```python
from build123d import *

# Parameters (mm, degrees)
SKETCH1_W           = 180
SKETCH1_H           = 180
SKETCH1_R           = 1.5
BOSS_EXTRUDE1_DEPTH = 5
CUT_EXTRUDE1_REACH  = 129.377
SKETCH4_W           = 5.1
SKETCH4_H           = 10
SKETCH4_W_2         = 10
SKETCH4_H_2         = 5.1
SKETCH4_W_3         = 125
SKETCH4_H_3         = 45
SKETCH5_R           = 1.55
CUT_EXTRUDE3_DEPTH  = 128.377392029
SKETCH6_W           = 4
SKETCH6_H           = 30
SKETCH6_R           = 1.3
CUT_EXTRUDE5_DEPTH  = 10
SKETCH7_R           = 1.55
CUT_EXTRUDE6_DEPTH  = 128.377392029
FILLET1_R           = 3


with BuildPart() as part:
    # Sketch1 → Boss-Extrude1 (new body)
    with BuildSketch(Plane(origin=(0, 0, 0), x_dir=(1, 0, 0), z_dir=(0, 1, 0))):
        Rectangle(SKETCH1_W, SKETCH1_H)
        with Locations(Location((-86, 86, 0), (0, 0, 270))):
            Circle(SKETCH1_R, mode=Mode.SUBTRACT)
        with Locations(Location((86, 86, 0), (0, 0, 270))):
            Circle(SKETCH1_R, mode=Mode.SUBTRACT)
        with Locations(Location((85.840740741, -86, 0), (0, 0, 270))):
            Circle(SKETCH1_R, mode=Mode.SUBTRACT)
        with Locations(Location((-86.159259259, -86, 0), (0, 0, 270))):
            Circle(SKETCH1_R, mode=Mode.SUBTRACT)
    extrude(amount=BOSS_EXTRUDE1_DEPTH)

    # Sketch4 → Cut-Extrude1 (cut, up to next)
    with BuildSketch(Plane(origin=(0, 5, 0), x_dir=(1, 0, 0), z_dir=(0, 1, 0)), mode=Mode.PRIVATE) as cut_extrude1_sk1:
        with Locations((67.45, -28.333333333)):
            Rectangle(SKETCH4_W, SKETCH4_H)
    cut_extrude1_tool1 = extrude(cut_extrude1_sk1.sketch, amount=-CUT_EXTRUDE1_REACH, mode=Mode.PRIVATE) & part.part
    # Sketch4 → Cut-Extrude1 (cut, up to next)
    with BuildSketch(Plane(origin=(0, 5, 0), x_dir=(1, 0, 0), z_dir=(0, 1, 0)), mode=Mode.PRIVATE) as cut_extrude1_sk2:
        with Locations((37.5, -12.55)):
            Rectangle(SKETCH4_W_2, SKETCH4_H_2)
    cut_extrude1_tool2 = extrude(cut_extrude1_sk2.sketch, amount=-CUT_EXTRUDE1_REACH, mode=Mode.PRIVATE) & part.part
    # Sketch4 → Cut-Extrude1 (cut, up to next)
    with BuildSketch(Plane(origin=(0, 5, 0), x_dir=(1, 0, 0), z_dir=(0, 1, 0)), mode=Mode.PRIVATE) as cut_extrude1_sk3:
        with Locations((0, -12.55)):
            Rectangle(SKETCH4_W_2, SKETCH4_H_2)
    cut_extrude1_tool3 = extrude(cut_extrude1_sk3.sketch, amount=-CUT_EXTRUDE1_REACH, mode=Mode.PRIVATE) & part.part
    # Sketch4 → Cut-Extrude1 (cut, up to next)
    with BuildSketch(Plane(origin=(0, 5, 0), x_dir=(1, 0, 0), z_dir=(0, 1, 0)), mode=Mode.PRIVATE) as cut_extrude1_sk4:
        with Locations((-37.5, -12.55)):
            Rectangle(SKETCH4_W_2, SKETCH4_H_2)
    cut_extrude1_tool4 = extrude(cut_extrude1_sk4.sketch, amount=-CUT_EXTRUDE1_REACH, mode=Mode.PRIVATE) & part.part
    # Sketch4 → Cut-Extrude1 (cut, up to next)
    with BuildSketch(Plane(origin=(0, 5, 0), x_dir=(1, 0, 0), z_dir=(0, 1, 0)), mode=Mode.PRIVATE) as cut_extrude1_sk5:
        with Locations((-67.45, -28.333333333)):
            Rectangle(SKETCH4_W, SKETCH4_H)
    cut_extrude1_tool5 = extrude(cut_extrude1_sk5.sketch, amount=-CUT_EXTRUDE1_REACH, mode=Mode.PRIVATE) & part.part
    # Sketch4 → Cut-Extrude1 (cut, up to next)
    with BuildSketch(Plane(origin=(0, 5, 0), x_dir=(1, 0, 0), z_dir=(0, 1, 0)), mode=Mode.PRIVATE) as cut_extrude1_sk6:
        with Locations((-37.5, -67.45)):
            Rectangle(SKETCH4_W_2, SKETCH4_H_2)
    cut_extrude1_tool6 = extrude(cut_extrude1_sk6.sketch, amount=-CUT_EXTRUDE1_REACH, mode=Mode.PRIVATE) & part.part
    # Sketch4 → Cut-Extrude1 (cut, up to next)
    with BuildSketch(Plane(origin=(0, 5, 0), x_dir=(1, 0, 0), z_dir=(0, 1, 0)), mode=Mode.PRIVATE) as cut_extrude1_sk7:
        with Locations((67.45, -51.666666667)):
            Rectangle(SKETCH4_W, SKETCH4_H)
    cut_extrude1_tool7 = extrude(cut_extrude1_sk7.sketch, amount=-CUT_EXTRUDE1_REACH, mode=Mode.PRIVATE) & part.part
    # Sketch4 → Cut-Extrude1 (cut, up to next)
    with BuildSketch(Plane(origin=(0, 5, 0), x_dir=(1, 0, 0), z_dir=(0, 1, 0)), mode=Mode.PRIVATE) as cut_extrude1_sk8:
        with Locations((37.5, -67.45)):
            Rectangle(SKETCH4_W_2, SKETCH4_H_2)
    cut_extrude1_tool8 = extrude(cut_extrude1_sk8.sketch, amount=-CUT_EXTRUDE1_REACH, mode=Mode.PRIVATE) & part.part
    # Sketch4 → Cut-Extrude1 (cut, up to next)
    with BuildSketch(Plane(origin=(0, 5, 0), x_dir=(1, 0, 0), z_dir=(0, 1, 0)), mode=Mode.PRIVATE) as cut_extrude1_sk9:
        with Locations((0, -67.45)):
            Rectangle(SKETCH4_W_2, SKETCH4_H_2)
    cut_extrude1_tool9 = extrude(cut_extrude1_sk9.sketch, amount=-CUT_EXTRUDE1_REACH, mode=Mode.PRIVATE) & part.part
    # Sketch4 → Cut-Extrude1 (cut, up to next)
    with BuildSketch(Plane(origin=(0, 5, 0), x_dir=(1, 0, 0), z_dir=(0, 1, 0)), mode=Mode.PRIVATE) as cut_extrude1_sk10:
        with Locations((-67.45, -51.666666667)):
            Rectangle(SKETCH4_W, SKETCH4_H)
    cut_extrude1_tool10 = extrude(cut_extrude1_sk10.sketch, amount=-CUT_EXTRUDE1_REACH, mode=Mode.PRIVATE) & part.part
    # Sketch4 → Cut-Extrude1 (cut, up to next)
    with BuildSketch(Plane(origin=(0, 5, 0), x_dir=(1, 0, 0), z_dir=(0, 1, 0)), mode=Mode.PRIVATE) as cut_extrude1_sk11:
        with Locations((0, -40)):
            Rectangle(SKETCH4_W_3, SKETCH4_H_3)
    cut_extrude1_tool11 = extrude(cut_extrude1_sk11.sketch, amount=-CUT_EXTRUDE1_REACH, mode=Mode.PRIVATE) & part.part
    add(cut_extrude1_tool1.solids().sort_by_distance((67.45, 5, 28.333333))[0], mode=Mode.SUBTRACT)
    add(cut_extrude1_tool2.solids().sort_by_distance((37.5, 5, 12.55))[0], mode=Mode.SUBTRACT)
    add(cut_extrude1_tool3.solids().sort_by_distance((0, 5, 12.55))[0], mode=Mode.SUBTRACT)
    add(cut_extrude1_tool4.solids().sort_by_distance((-37.5, 5, 12.55))[0], mode=Mode.SUBTRACT)
    add(cut_extrude1_tool5.solids().sort_by_distance((-67.45, 5, 28.333333))[0], mode=Mode.SUBTRACT)
    add(cut_extrude1_tool6.solids().sort_by_distance((-37.5, 5, 67.45))[0], mode=Mode.SUBTRACT)
    add(cut_extrude1_tool7.solids().sort_by_distance((67.45, 5, 51.666667))[0], mode=Mode.SUBTRACT)
    add(cut_extrude1_tool8.solids().sort_by_distance((37.5, 5, 67.45))[0], mode=Mode.SUBTRACT)
    add(cut_extrude1_tool9.solids().sort_by_distance((0, 5, 67.45))[0], mode=Mode.SUBTRACT)
    add(cut_extrude1_tool10.solids().sort_by_distance((-67.45, 5, 51.666667))[0], mode=Mode.SUBTRACT)
    add(cut_extrude1_tool11.solids().sort_by_distance((0, 5, 40))[0], mode=Mode.SUBTRACT)

    # Sketch5 → Cut-Extrude3 (cut, through all)
    with BuildSketch(Plane(origin=(0, 5, 0), x_dir=(1, 0, 0), z_dir=(0, 1, 0))):
        with Locations(Location((-47, 52, 0), (0, 0, 270))):
            Circle(SKETCH5_R)
        with Locations(Location((-23, 52, 0), (0, 0, 270))):
            Circle(SKETCH5_R)
        with Locations(Location((-23, 28, 0), (0, 0, 270))):
            Circle(SKETCH5_R)
        with Locations(Location((-47, 28, 0), (0, 0, 270))):
            Circle(SKETCH5_R)
    extrude(amount=-CUT_EXTRUDE3_DEPTH, mode=Mode.SUBTRACT)

    # Sketch6 → Cut-Extrude5 (cut)
    with BuildSketch(Plane(origin=(0, 5, 0), x_dir=(1, 0, 0), z_dir=(0, 1, 0))):
        with Locations((18.75, 40)):
            Rectangle(SKETCH6_W, SKETCH6_H)
        with Locations((58, 40)):
            Rectangle(SKETCH6_W, SKETCH6_H)
        with Locations(Location((58, 60.125, 0), (0, 0, 270))):
            Circle(SKETCH6_R)
        with Locations(Location((18.75, 60.125, 0), (0, 0, 270))):
            Circle(SKETCH6_R)
        with Locations(Location((18.75, 19.875, 0), (0, 0, 270))):
            Circle(SKETCH6_R)
        with Locations(Location((58, 19.875, 0), (0, 0, 270))):
            Circle(SKETCH6_R)
    extrude(amount=-CUT_EXTRUDE5_DEPTH, mode=Mode.SUBTRACT)

    # Sketch7 → Cut-Extrude6 (cut, through all)
    with BuildSketch(Plane(origin=(0, 5, 0), x_dir=(1, 0, 0), z_dir=(0, 1, 0))):
        with Locations(Location((-77, -10, 0), (0, 0, 270))):
            Circle(SKETCH7_R)
        with Locations(Location((-77, -29, 0), (0, 0, 270))):
            Circle(SKETCH7_R)
        with Locations(Location((-77, -51, 0), (0, 0, 90))):
            Circle(SKETCH7_R)
        with Locations(Location((-77, -70, 0), (0, 0, 90))):
            Circle(SKETCH7_R)
        with Locations(Location((77, -29, 0), (0, 0, 90))):
            Circle(SKETCH7_R)
        with Locations(Location((77, -10, 0), (0, 0, 90))):
            Circle(SKETCH7_R)
        with Locations(Location((77, -70, 0), (0, 0, 270))):
            Circle(SKETCH7_R)
        with Locations(Location((77, -51, 0), (0, 0, 270))):
            Circle(SKETCH7_R)
    extrude(amount=-CUT_EXTRUDE6_DEPTH, mode=Mode.SUBTRACT)

    # Fillet1
    fillet1_edges = [part.edges().sort_by_distance(p)[0] for p in [
        (-90, 2.5, 90),
        (-90, 2.5, -90),
        (90, 2.5, -90),
        (90, 2.5, 90),
    ]]
    fillet(fillet1_edges, radius=FILLET1_R)


solid = part.part
```
Input: part model. Units: mm. Frame: model coordinates. A direction names the side the tool comes from. Coordinates: 2 decimals unless noted, no trailing zeros. Write each loop counter-clockwise with the first axis right and the second up, starting at its lowest first coordinate (ties: lowest second). Pieces come first, ordered by that corner, then holes. Notation, with made-up numbers: (-12.5, -27.5) - (14.5, -27.5) arc R31 cw to (14.5, 3.5) - close; hole circle Ø5 at (0.25, -3.75). An arc over 180 degrees is marked (long way). Put each result on its own line as item: value. Start each with the question number.
1) Reachability of faces 4 (the face through (90, 2, 1)), 5 (the face through (-1, 3, 17.5)) from +Z, -Z, +X, -X, +Y, -Y: full face, straight path, thin tool, end or side. Return the list, or none.
2) Cut plane A-A (x = -8). Return the cut outline in (y, z).
3) Mould query, pull axis X, two halves, no side actions, for faces 1 (the face through (-1, 2, 90)), 2 (the face through (-90, 2, 1)), 3 (the face through (-67, 3, 56.667)). Classes: pulls with the +X half, pulls with the -X half, needs draft (parallel to the pull), parting line crosses it, or undercut.
4) Cut plane B-B (x = -39). Return the cut outline in (y, z).
5) Ray query, L1, parallel to X at y = 3, z = -49; L2, parallel to X at y = 2.25, z = -52; L3, parallel to Z at x = 77, y = 3.45. Return the intervals inside material, ascending.
6) Contact query for flat-ended pins moving along their axis: pin 1 (5 mm diameter, centred on x = -47, z = -52, fed in from -Y); pin 2 (2.5 mm diameter, centred on x = -77, z = 29, fed in from -Y). Output: stop coordinate, or through.
7) Cut plane C-C (y = 1.55). State how many separate pieces and enclosed holes the cut face has, plus the area to 3 significant figures.
Resolved:
1. face 4: +Z, -Z, +X, +Y, -Y
1. face 5: +Y, -Y
2. outline: (0, -90) - (5, -90) - (5, 17.5) - (0, 17.5) - close; (0, 62.5) - (5, 62.5) - (5, 90) - (0, 90) - close
3. face 1: needs draft
3. face 2: pulls with the -X half
3. face 3: undercut
4. outline: (0, -90) - (5, -90) - (5, 10) - (0, 10) - close; (0, 15.1) - (5, 15.1) - (5, 17.5) - (0, 17.5) - close; (0, 62.5) - (5, 62.5) - (5, 64.9) - (0, 64.9) - close; (0, 70) - (5, 70) - (5, 90) - (0, 90) - close
5. L1: x = -90 to 16.75, 20.75 to 56, 60 to 90
5. L2: x = -90 to -48.55, -45.45 to -24.55, -21.45 to 16.75, 20.75 to 56, 60 to 90
5. L3: z = -90 to 8.45, 11.55 to 27.45, 30.55 to 49.45, 52.55 to 68.45, 71.55 to 90
6. pin 1: stops at y = 0
6. pin 2: passes through
7. separate pieces: 1
7. enclosed holes: 33
7. area: 25,900 mm2
